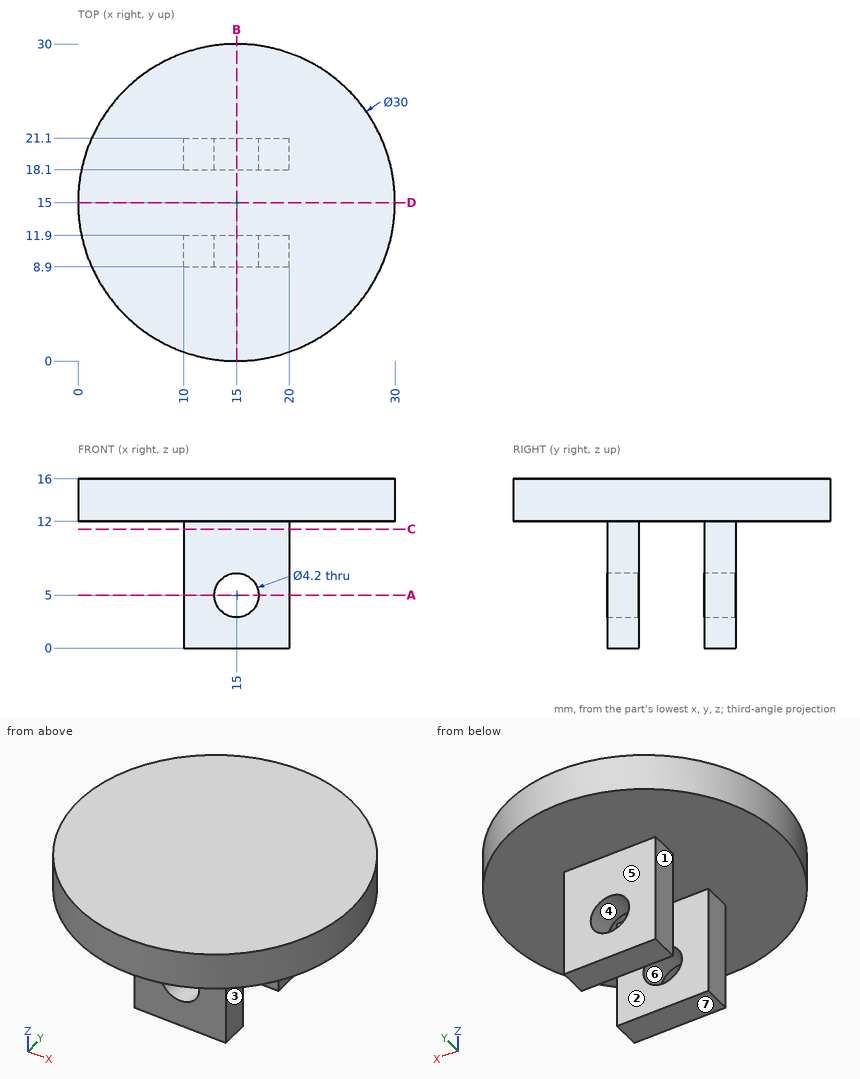
Study the drawing (mm; zero at the part's minimum x, y, z) and answer. A direction names the side the tool comes from. Give positions to 0.01 mm unless a question says otherwise; leave off trailing zeros. Order: outer loops, then holes, each group sorted by start corner. A loop starts at its lowest first (then second) coordinate and runs counter-clockwise, first axis right, second up. Notation, with made-up numbers: (4, 47) - (55, 47) arc R8 cw to (55, 51) - close; hole circle Ø1 at (45, -20.75). An arc over 180 degrees is marked (long way). Use one line per item in the form item = value. Start each with the question number.
(1) Flat-ended cylindrical pins translate along their axes: pin 1 Ø2.5 at (y, z) = (9.5, 5.5) entering from +X; pin 2 Ø6 at (y, z) = (19, 2) entering from -X; pin 3 Ø5.5 at (x, z) = (15, 5) entering from +Y; pin 4 Ø15 at (x, y) = (9, 11) entering from -Z. Find the tip coordinate at first contact, or state that the pin passes through.
(2) For the marked faces 1, 2 and 3, determine the directions among +Z, -Z, +X, -X, +Y, -Y from which every point of the face is accessible in a straight line to the end or side of a thin tool.
(3) Consider line 1 (X direction, y = 11.1, z = 5); line 2 (Y direction, x = 11.5, z = 11.75); line 3 (Z direction, x = 14.25, y = 16.25). Determine where each line is inside the solid, lowest interval first. Write a range as from..to.
(4) A cutting plane is placed at D-D, the plane y = 15. Write down the section's boundary in (x, z).
(5) A cutting plane is placed at A-A, the plane z = 5. Write down the section's boundary in (x, y), then the cut area to 3 significant figures.
(6) The mould has two halves that part along Z. Classify the marked faces 4, 5, 6 and 7: released by +Z, released by -Z, zero draft, split by the parting line, or undercut.
(7) A cutting plane is placed at C-C, the plane z = 11.25. Write down the section's boundary in (x, y).
(8) A cutting plane is placed at B-B, the plane x = 15. Write down the section's boundary in (y, z).
Ans:
q1.pin_1 = 20
q1.pin_2 = 10
q1.pin_3 = 21.1
q1.pin_4 = 0
q2.face_1 = -Z, -X, +Y, -Y
q2.face_2 = -Z, +X, -X
q2.face_3 = -Z, +X, +Y, -Y
q3.line_1 = 10..12.9, 17.1..20
q3.line_2 = 8.9..11.9, 18.1..21.1
q3.line_3 = 12..16
q4.outline = (0, 12) - (30, 12) - (30, 16) - (0, 16) - close
q5.outline = (10, 8.9) - (12.9, 8.9) - (12.9, 11.9) - (10, 11.9) - close; (10, 18.1) - (12.9, 18.1) - (12.9, 21.1) - (10, 21.1) - close; (17.1, 8.9) - (20, 8.9) - (20, 11.9) - (17.1, 11.9) - close; (17.1, 18.1) - (20, 18.1) - (20, 21.1) - (17.1, 21.1) - close
q5.area = 34.8 mm^2
q6.face_4 = undercut
q6.face_5 = zero draft
q6.face_6 = undercut
q6.face_7 = released by -Z
q7.outline = (10, 8.9) - (20, 8.9) - (20, 11.9) - (10, 11.9) - close; (10, 18.1) - (20, 18.1) - (20, 21.1) - (10, 21.1) - close
q8.outline = (0, 12) - (8.9, 12) - (8.9, 7.1) - (11.9, 7.1) - (11.9, 12) - (18.1, 12) - (18.1, 7.1) - (21.1, 7.1) - (21.1, 12) - (30, 12) - (30, 16) - (0, 16) - close; (8.9, 0) - (11.9, 0) - (11.9, 2.9) - (8.9, 2.9) - close; (18.1, 0) - (21.1, 0) - (21.1, 2.9) - (18.1, 2.9) - close
